from build123d import *

# Parameters (mm, degrees)
SKETCH_2_R      = 2.1
EXTRUDE_1_DEPTH = 3


with BuildPart() as part:
    # 草图2 → 凸台-拉伸1 (new body)
    with BuildSketch(Plane.ZY.offset(116.606649797)):
        with BuildLine():
            Line((1030.654259328, -102.283530386), (1082.654259328, -102.283530386))
            Line((1082.654259328, -102.283530386), (1082.654259328, -93.783530386))
            Line((1082.654259328, -93.783530386), (1087.154259328, -93.783530386))
            Line((1087.154259328, -93.783530386), (1087.154259328, -63.783530386))
            Line((1087.154259328, -63.783530386), (1087.154259328, -53.200711014))
            ThreePointArc((1087.154259328, -53.200711014), (1056.654259328, -35.273255635), (1026.154259328, -53.200711014))
            Line((1026.154259328, -53.200711014), (1026.154259328, -63.783530386))
            Line((1026.154259328, -63.783530386), (1026.154259328, -111.416059373))
            Line((1026.154259328, -111.416059373), (1030.654259328, -111.416059373))
            Line((1030.654259328, -111.416059373), (1030.654259328, -102.283530386))
        make_face()
        with Locations(Location((1074.154259328, -81.283530386, 0), (0, 0, 270))):
            Circle(SKETCH_2_R, mode=Mode.SUBTRACT)
        with Locations(Location((1039.154259328, -81.283530386, 0), (0, 0, 270))):
            Circle(SKETCH_2_R, mode=Mode.SUBTRACT)
        with Locations(Location((1074.154259328, -46.283530386, 0), (0, 0, 270))):
            Circle(SKETCH_2_R, mode=Mode.SUBTRACT)
        with Locations(Location((1039.154259328, -46.283530386, 0), (0, 0, 270))):
            Circle(SKETCH_2_R, mode=Mode.SUBTRACT)
    extrude(amount=EXTRUDE_1_DEPTH)


solid = part.part
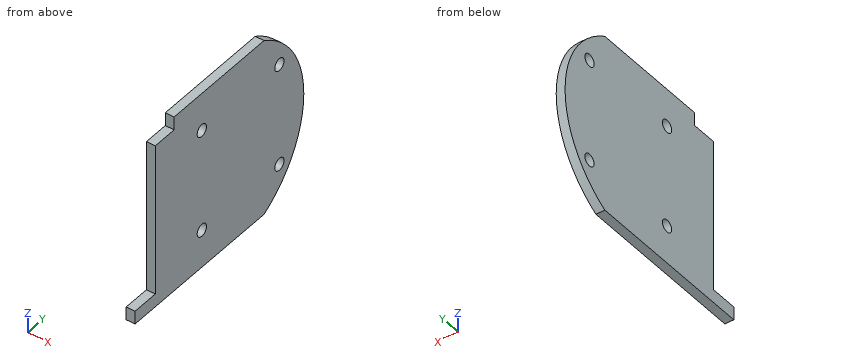
For this review, take the finished solid that the model builds, in its own axes (mm). Give positions to 0.01 mm unless a question says otherwise; leave off trailing zeros. Loops run counter-clockwise (first coordinate to the right, second up) from the corner with the lowest first, then second, coordinate; pieces in that order, holes last. Notation, with made-up numbers: M 31.5,81.25 L 62.5,81.25 A21 cw 62.5,94.25 Z; hole C 44.5,66 d5. An arc over 180 degrees is marked long. Answer as a JSON object with one key per item and string values. Group by question number.
Q1. Add section A-A on y = -45. Give the boundary of the cut face in (x, z), and give its area (3 significant figures).
Q2. Add section C-C on z = 1033.5. Give the boundary of the cut face in (x, y).
Q3. Insertion check: P1, Ø0.9, axis at x = -118.5, y = -108, coming from the +Z side; P2, Ø3.5, axis at y = -81.28, z = 1074.15, coming from the +X side; P3, Ø0.9, axis at x = -118.5, y = -98, coming from the +Z side; P4, Ø1.5, axis at x = -118, z = 1085, coming from the -Y side. Each pin has a flat end and moves straight along its axis. Give the tip position at first contact, or say it passes through.
Q4. Add section B-B on x = -117.75. Give the boundary of the cut face in (y, z), and give its area (3 significant figures).
Q5. Add section D-D on y = -95. Give the boundary of the cut face in (x, z), and give its area (4 significant figures).
Q6. For probe 1 along Y at (x, z) = (-119.25, 1076); probe 2 along Y at (x, z) = (-117.95, 1073); probe 3 along Z at (x, y) = (-117.3, -46), list the stretches that pass through material, from the lowest coordinate up. Write a range as [from, to].
Checked values:
{
 "1": {"outline": "M -119.61,1032.48 L -116.61,1032.48 L -116.61,1037.49 L -119.61,1037.49 Z; M -119.61,1040.82 L -116.61,1040.82 L -116.61,1072.49 L -119.61,1072.49 Z; M -119.61,1075.82 L -116.61,1075.82 L -116.61,1080.83 L -119.61,1080.83 Z", "area": "125 mm²"},
 "2": {"outline": "M -119.61,-102.28 L -116.61,-102.28 L -116.61,-44.06 L -119.61,-44.06 Z"},
 "3": {"P1": "z = 1030.65", "P2": "through", "P3": "z = 1082.65", "P4": "y = -93.78"},
 "4": {"outline": "M -111.42,1026.15 L -53.2,1026.15 A34.91 ccw -53.2,1087.15 L -93.78,1087.15 L -93.78,1082.65 L -102.28,1082.65 L -102.28,1030.65 L -111.42,1030.65 Z; hole C -81.28,1039.15 d4.2; hole C -81.28,1074.15 d4.2; hole C -46.28,1039.15 d4.2; hole C -46.28,1074.15 d4.2", "area": "3,720 mm²"},
 "5": {"outline": "M -119.61,1026.15 L -116.61,1026.15 L -116.61,1082.65 L -119.61,1082.65 Z", "area": "169.5 mm²"},
 "6": {"probe 1": "[-102.28, -82.29], [-80.28, -47.29], [-45.28, -41.12]", "probe 2": "[-102.28, -83.04], [-79.53, -48.04], [-44.53, -39.34]", "probe 3": "[1031.48, 1037.07], [1041.24, 1072.07], [1076.24, 1081.83]"}
}
